For this review, take the finished solid that the model builds, in its own axes (mm). A direction names the side the tool comes from. Coordinates: 2 decimals unless noted, no trailing zeros. Order: outer loops, then holes, each group sorted by start corner. A loop starts at its lowest first (then second) coordinate and runs counter-clockwise, first axis right, second up. Notation, with made-up numbers: (-23, 22.5) - (8, 22.5) arc R3 ccw to (8, 27.5) - close; hole circle Ø5 at (17.25, 29). An arc over 180 degrees is marked (long way). One line per item, written item: value. Start each with the question number.
(1) Consider section D-D on x = 7.5. Write out the cut boundary in (y, z), then the cut area to 3 significant figures.
(2) Mouldability with a two-part tool opening along X and no side actions: class faces 1 (the flat face through (0, 8, -27)), 2 (the cylindrical face through (11.5, 4.93, -21.77)), 3 (the flat face through (15, 14, -54)) as released by +X, released by -X, zero draft, split by the parting line, or undercut.
(3) For faces 4 (the flat face through (10, 15, -7)), 5 (the flat face through (10, 18, -4)), 6 (the flat face through (15, 14, -1)), 7 (the flat face through (17, 4, -7)), list the 3-axis set-ups (+Z, -Z, +X, -X, +Y, -Y) from which the entire face can be reached by the end or side of a thin tool; tool diameter is ignored.
(4) Consider section A-A on z = -49.5. Write out the cut boundary in (x, y), then the cut area to 3 significant figures.
(5) Consider section B-B on x = 17. Write out the cut boundary in (y, z), then the cut area to 3 significant figures.
(6) Clearance check with flat-ended pins moving along their axes: pin 1 (1.2 mm diameter, centred on x = 13.5, z = -54.5, fed in from -Y); pin 2 (1.2 mm diameter, centred on x = 17, y = 4, fed in from -Z); pin 3 (0.6 mm diameter, centred on x = 15, z = -2.5, fed in from +Y). State where each tip first meets the part, or that it passes through.
(7) To check wall thickness, follow line 1 along X through (y, z) = (17.6, -2.4); line 2 along X through (y, z) = (4, -4.75); line 3 along Y through (x, z) = (3, -50.2). State the ranges of each line that lie inside material, in increasing order.
(8) Consider section C-C on z = -18.5. Write out the cut boundary in (x, y).
```python
from build123d import *

# Parameters (mm, degrees)
SKETCH_1_W          = 20
SKETCH_1_H          = 55
EXTRUDE_1_DEPTH     = 20
SKETCH_2_W          = 20
SKETCH_2_H          = 41
CUT_EXTRUDE_1_DEPTH = 10
SKETCH_3_W          = 2.8
SKETCH_3_H          = 55
CUT_EXTRUDE_2_DEPTH = 2
SKETCH_4_R          = 1
CUT_EXTRUDE_3_DEPTH = 4
SKETCH_5_R          = 5
CUT_EXTRUDE_4_DEPTH = 62.846584384
SKETCH_6_R          = 1
CUT_EXTRUDE_5_DEPTH = 7
CUT_EXTRUDE_START   = -7
SKETCH_7_R          = 1
CUT_EXTRUDE_6_DEPTH = 7
CUT_EXTRUDE_7_DEPTH = 1.5
CUT_EXTRUDE_START_2 = -1.5
CUT_EXTRUDE_8_DEPTH = 1.5


with BuildPart() as part:
    # Эскиз1 → Бобышка-Вытянуть1 (new body)
    with BuildSketch(Plane(origin=(0, 0, 0), x_dir=(1, 0, 0), z_dir=(0, 1, 0))):
        with Locations((10, 27.5)):
            Rectangle(SKETCH_1_W, SKETCH_1_H)
    extrude(amount=EXTRUDE_1_DEPTH)

    # Эскиз2 → Вырез-Вытянуть1 (cut)
    with BuildSketch(Plane(origin=(0, 20, 0), x_dir=(1, 0, 0), z_dir=(0, 1, 0))):
        with Locations((10, 27.5)):
            Rectangle(SKETCH_2_W, SKETCH_2_H)
    extrude(amount=-CUT_EXTRUDE_1_DEPTH, mode=Mode.SUBTRACT)

    # Эскиз3 → Вырез-Вытянуть2 (cut)
    with BuildSketch(Plane(origin=(0, 20, 0), x_dir=(1, 0, 0), z_dir=(0, 1, 0))):
        with Locations((10, 27.5)):
            Rectangle(SKETCH_3_W, SKETCH_3_H)
    extrude(amount=-CUT_EXTRUDE_2_DEPTH, mode=Mode.SUBTRACT)

    # Эскиз4 → Вырез-Вытянуть3 (cut)
    with BuildSketch(Plane(origin=(0, 20, 0), x_dir=(1, 0, 0), z_dir=(0, 1, 0))):
        with Locations(Location((15, 52.6, 0), (0, 0, 270))):
            Circle(SKETCH_4_R)
        with Locations(Location((5, 52.6, 0), (0, 0, 270))):
            Circle(SKETCH_4_R)
        with Locations(Location((15, 2.4, 0), (0, 0, 270))):
            Circle(SKETCH_4_R)
        with Locations(Location((5, 2.4, 0), (0, 0, 270))):
            Circle(SKETCH_4_R)
    extrude(amount=-CUT_EXTRUDE_3_DEPTH, mode=Mode.SUBTRACT)

    # Эскиз5 → Вырез-Вытянуть4 (cut, through all)
    with BuildSketch(Plane.XZ):
        with Locations(Location((10, -17, 0), (0, 0, 270))):
            Circle(SKETCH_5_R)
        with Locations(Location((10, -30, 0), (0, 0, 270))):
            Circle(SKETCH_5_R)
    extrude(amount=-CUT_EXTRUDE_4_DEPTH, mode=Mode.SUBTRACT)

    # Эскиз6 → Вырез-Вытянуть5 (cut)
    with BuildSketch(Plane(origin=(0, 0, -55), x_dir=(-1, 0, 0), z_dir=(0, 0, -1))):
        with Locations((-17, 4)):
            Circle(SKETCH_6_R)
        with Locations((-3, 4)):
            Circle(SKETCH_6_R)
    extrude(amount=-CUT_EXTRUDE_5_DEPTH, mode=Mode.SUBTRACT)

    # Эскиз7 → Вырез-Вытянуть6 (cut)
    with BuildSketch(Plane.XY.offset(CUT_EXTRUDE_START)):
        with Locations(Location((3, 4, 0), (0, 0, 180))):
            Circle(SKETCH_7_R)
        with Locations(Location((17, 4, 0), (0, 0, 180))):
            Circle(SKETCH_7_R)
    extrude(amount=CUT_EXTRUDE_6_DEPTH, mode=Mode.SUBTRACT)

    # Эскиз8 → Вырез-Вытянуть7 (cut)
    with BuildSketch(Plane(origin=(0, 0, -55), x_dir=(-1, 0, 0), z_dir=(0, 0, -1))):
        with BuildLine():
            Line((-10, 14), (-20, 14))
            Line((-20, 14), (-20, 0))
            Line((-20, 0), (0, 0))
            Line((0, 0), (0, 4))
            ThreePointArc((0, 4), (-2.928932188, 11.071067812), (-10, 14))
        make_face()
    extrude(amount=-CUT_EXTRUDE_7_DEPTH, mode=Mode.SUBTRACT)

    # Эскиз9 → Вырез-Вытянуть8 (cut)
    with BuildSketch(Plane.XY.offset(CUT_EXTRUDE_START_2)):
        with BuildLine():
            Line((0, 4), (0, 0))
            Line((0, 0), (20, 0))
            Line((20, 0), (20, 14))
            Line((20, 14), (10, 14))
            ThreePointArc((10, 14), (2.928932188, 11.071067812), (0, 4))
        make_face()
    extrude(amount=CUT_EXTRUDE_8_DEPTH, mode=Mode.SUBTRACT)


solid = part.part
```
Geometry check:
1. outline: (0, -53.5) - (13.68, -53.5) - (13.68, -55) - (20, -55) - (20, -48) - (10, -48) - (10, -34.33) - (0, -34.33) - close; (0, -25.67) - (10, -25.67) - (10, -21.33) - (0, -21.33) - close; (0, -12.67) - (10, -12.67) - (10, -7) - (20, -7) - (20, 0) - (13.68, 0) - (13.68, -1.5) - (0, -1.5) - close
1. area: 476 mm^2
2. face 1: released by -X
2. face 2: undercut
2. face 3: zero draft
3. face 4: +X, -X, +Y
3. face 5: +Z, -Z, +Y
3. face 6: +Z, +X, -Y
3. face 7: +Z
4. outline: (0, 0) - (20, 0) - (20, 20) - (11.4, 20) - (11.4, 18) - (8.6, 18) - (8.6, 20) - (0, 20) - close; hole circle Ø2 at (3, 4); hole circle Ø2 at (17, 4)
4. area: 388 mm^2
5. outline: (0, -53.5) - (3, -53.5) - (3, -48) - (5, -48) - (5, -53.5) - (14, -53.5) - (14, -55) - (20, -55) - (20, -48) - (10, -48) - (10, -7) - (20, -7) - (20, 0) - (14, 0) - (14, -1.5) - (5, -1.5) - (5, -7) - (3, -7) - (3, -1.5) - (0, -1.5) - close
5. area: 626 mm^2
6. pin 1: stops at y = 14
6. pin 2: stops at z = -48
6. pin 3: stops at y = 16
7. line 1: x = 0 to 4, 6 to 14, 16 to 20
7. line 2: x = 0 to 2, 4 to 16, 18 to 20
7. line 3: y = 0 to 3, 5 to 20
8. outline: (0, 0) - (5.23, 0) - (5.23, 10) - (0, 10) - close; (14.77, 0) - (20, 0) - (20, 10) - (14.77, 10) - close
